Could you check a few things on this model? Use its own coordinates, in mm. Face numbers are marked on the shaded views. A direction names the side the tool comes from. Give positions to 0.01 mm unless a question says otherwise; leave off trailing zeros. Loops run counter-clockwise (first coordinate to the right, second up) from the corner with the lowest first, then second, coordinate; pieces in that order, holes last. Notation, with made-up numbers: M 79,63 L 112,63 A22 ccw 112,99 Z; hole C 2,-34.5 d3. An arc over 180 degrees is marked long. Use CSV: the item, a comma, the result in double quotes.
```python
from build123d import *

# Parameters (mm, degrees)
SKETCH_1_R          = 2
EXTRUDE_1_DEPTH     = 20
SKETCH_2_W          = 18
SKETCH_2_H          = 18
CUT_EXTRUDE_1_DEPTH = 227.406099505


with BuildPart() as part:
    # 草图1 → 凸台-拉伸1 (new body)
    with BuildSketch(Plane(origin=(0, 0, 0), x_dir=(1, 0, 0), z_dir=(0, 1, 0))):
        Polygon((98.036220612, 64.925160964), (98.036220612, 41.831150196), (-87.17089272, -65.098226542), (-97.17089272, -47.777718466), align=None)
        with Locations(Location((-83.481517274, -51.486680212, 0), (0, 0, 270))):
            Circle(SKETCH_1_R, mode=Mode.SUBTRACT)
        with Locations(Location((-66.161009198, -41.486680212, 0), (0, 0, 270))):
            Circle(SKETCH_1_R, mode=Mode.SUBTRACT)
        with Locations(Location((-48.86962253, -31.437972504, 0), (0, 0, 270))):
            Circle(SKETCH_1_R, mode=Mode.SUBTRACT)
        with Locations(Location((-40.209368493, -26.437972504, 0), (0, 0, 270))):
            Circle(SKETCH_1_R, mode=Mode.SUBTRACT)
        with Locations(Location((-31.549114455, -21.437972504, 0), (0, 0, 270))):
            Circle(SKETCH_1_R, mode=Mode.SUBTRACT)
        with Locations(Location((72.055458499, 38.37815558, 0), (0, 0, 270))):
            Circle(SKETCH_1_R, mode=Mode.SUBTRACT)
        with Locations(Location((85.045839556, 45.87815558, 0), (0, 0, 270))):
            Circle(SKETCH_1_R, mode=Mode.SUBTRACT)
    extrude(amount=EXTRUDE_1_DEPTH)

    # 草图2 → 切除-拉伸1 (cut, through all)
    with BuildSketch(Plane(origin=(-93.566528503, 0, 54.020660418), x_dir=(0.500000000000001, 0, 0.8660254037844382), z_dir=(-0.866025403784438, 0, 0.5000000000000009))):
        with Locations((2.791271567, 10)):
            Rectangle(SKETCH_2_W, SKETCH_2_H)
    extrude(amount=-CUT_EXTRUDE_1_DEPTH, mode=Mode.SUBTRACT)


solid = part.part
```
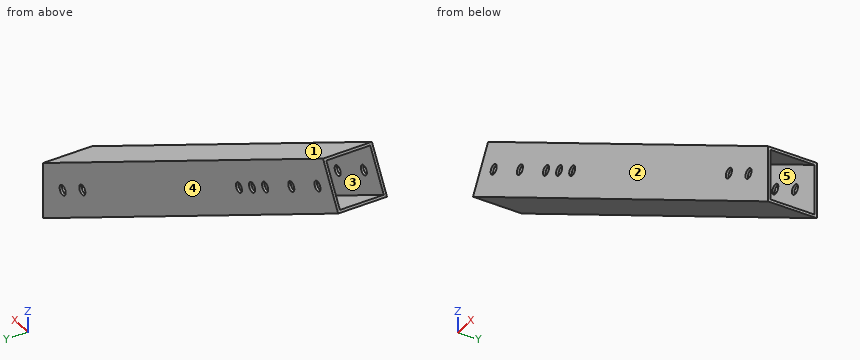
1. If we mould it in two halves opening along X, with no side actions, what happens to the marked faces 1, 2 and 3? For each: +X half, -X half, draft (parallel to the pull), parting line (faces both ways), or undercut.
Outcome:
face 1,"+X half"
face 2,"draft"
face 3,"undercut"
2. I want a section at B-B, the plane z = 14. List the corners of the cut face in (x, y) for me, then the cut area to 3 significant figures.
Outcome:
outline,"M -38.67,0 L 1.33,0 L 1.33,20 L -38.67,20 Z; hole M -36.67,1 L -0.67,1 L -0.67,19 L -36.67,19 Z"
area,"152 mm2"
3. I want a section at A-A, the plane y = 13.25. List the corners of the cut face in (x, z) for me, then the cut area to 3 significant figures.
Outcome:
outline,"M -97.17,47.78 L 98.04,-64.93 L 98.04,-63.77 L -96.67,48.64 Z; M -87.67,64.23 L 98.04,-42.99 L 98.04,-41.83 L -87.17,65.1 Z"
area,"439 mm2"
4. I'm going to push flat-ended pins straight in: pin 1 Ø1 at (x, y) = (-68, 3.5) entering from +Z; pin 2 Ø2 at (y, z) = (13.5, -5) entering from -X; pin 3 Ø3 at (x, z) = (85.05, -45.88) entering from -Y; pin 4 Ø1 at (y, z) = (18, 47) entering from +X. Where does each tip first touch, or does it pass through?
Outcome:
pin 1,"z = 54.32"
pin 2,"x = -7.49"
pin 3,"through"
pin 4,"x = -54.96"
5. I want a section at D-D, the plane x = -73. List the corners of the cut face in (y, z) for me.
Outcome:
outline,"M 0,33.82 L 20,33.82 L 20,56.92 L 0,56.92 Z; hole M 1,34.98 L 19,34.98 L 19,55.76 L 1,55.76 Z"
6. Please list where these lines run through material, in increasing order: line 1 (Y direction, x = -29.5, z = 26.5); line 2 (Z direction, x = -81, y = 18.5); line 3 (X direction, y = 13.25, z = 8.5).
Outcome:
line 1,"0 to 1, 19 to 20"
line 2,"38.44 to 39.6, 60.38 to 61.54"
line 3,"-29.14 to -27.14, 8.86 to 10.86"
7. Which directions (+Z, -Z, +X, -X, +Y, -Y) give clear straight access to the entire face, cutting with the end or side of a thin tool? Please do the marked faces 4 and 5.
Outcome:
face 4,"+Z, -Z, +X, -X, +Y"
face 5,"none"
8. I want a section at C-C, the plane z = -50. List the corners of the cut face in (x, y) for me, then the cut area to 3 significant figures.
Outcome:
outline,"M 72.19,0 L 98.04,0 L 98.04,1 L 74.19,1 L 74.19,19 L 98.04,19 L 98.04,20 L 72.19,20 Z"
area,"87.7 mm2"
